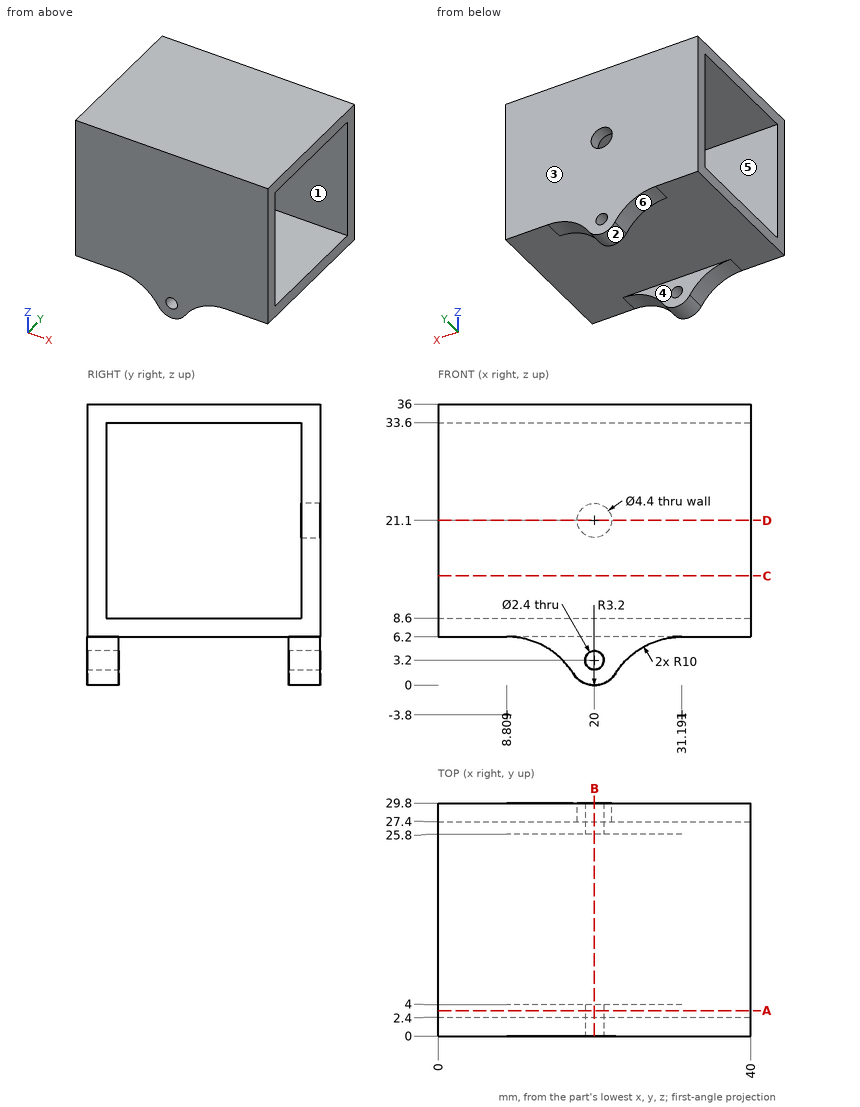
Answer from the drawing. Dimensions are ordinates in mm from the lowest x, y and z of the part. A direction names the side the tool comes from. Coordinates: 2 decimals unless noted, no trailing zeros. Write each loop counter-clockwise with the first axis right and the second up, starting at its lowest first coordinate (ties: lowest second). Pieces come first, ordered by that corner, then holes. Notation, with made-up numbers: M -33,48.25 L -3,48.25 A13 ccw -3,65.25 Z; hole C -8.5,-14.75 d8. An arc over 180 degrees is marked long. Use one line per item in the form item = value. Start each with the question number.
1. The part is cut by section A-A (y = 3.25). Give the vertices of the cut face in (x, z), plus the area to 3 significant figures.
2. Straight lines are drawn through the part: probe 1 along Z at (x, y) = (20, 27.2); probe 2 along Z at (x, y) = (16, 16.25); probe 3 along X at (y, z) = (29.05, 21.1). For each, find the intervals that lie inside material, in ascending order. Write a range as from..to.
3. The part is cut by section B-B (x = 20). Give the vertices of the cut face in (y, z), plus the area to 3 significant figures.
4. The part is cut by section C-C (z = 14). Give the vertices of the cut face in (x, y), plus the area to 3 significant figures.
5. A tool of negligible diameter and unlimited length cuts with its end or side. For the marked faces 5 and 6, from which of +Z, -Z, +X, -X, +Y, -Y can it reach the whole face along a straight path? Write none if from no direction.
6. The mould has two halves that part along Y. Classify the marked faces 1, 2, 3 and 4: released by +Y, released by -Y, zero draft, split by the parting line, or undercut.
7. Each of these flat-tipped pins is pushed along its axis until it touches: P1, Ø5, axis at x = 19, z = 25.5, coming from the -Y side; P2, Ø7.5, axis at x = 17, y = 12.5, coming from the -Z side; P3, Ø2, axis at x = 20, z = 3.2, coming from the +Y side. Where does it stop, or does it pass through?
8. The part is cut by section D-D (z = 21.1). Give the vertices of the cut face in (x, y), plus the area to 3 significant figures.
Evaluation:
q1.outline = M 0,6.2 L 8.81,6.2 A10 cw 17.29,1.5 A3.2 ccw 22.71,1.5 A10 cw 31.19,6.2 L 40,6.2 L 40,8.6 L 0,8.6 Z; M 0,33.6 L 40,33.6 L 40,36 L 0,36 Z; hole C 20,3.2 d2.4
q1.area = 242 mm^2
q2.probe_1 = 0..2, 4.4..8.6, 33.6..36
q2.probe_2 = 6.2..8.6, 33.6..36
q2.probe_3 = 0..17.8, 22.2..40
q3.outline = M 0,0 L 4,0 L 4,2 L 0,2 Z; M 0,4.4 L 4,4.4 L 4,6.2 L 25.8,6.2 L 25.8,4.4 L 29.8,4.4 L 29.8,18.9 L 27.4,18.9 L 27.4,8.6 L 2.4,8.6 L 2.4,33.6 L 27.4,33.6 L 27.4,23.3 L 29.8,23.3 L 29.8,36 L 0,36 Z; M 25.8,0 L 29.8,0 L 29.8,2 L 25.8,2 Z
q3.area = 283 mm^2
q4.outline = M 0,0 L 40,0 L 40,2.4 L 0,2.4 Z; M 0,27.4 L 40,27.4 L 40,29.8 L 0,29.8 Z
q4.area = 192 mm^2
q5.face_5 = +X, -X
q5.face_6 = -Z, -X, +Y, -Y
q6.face_1 = undercut
q6.face_2 = zero draft
q6.face_3 = released by +Y
q6.face_4 = undercut
q7.P1 = 0
q7.P2 = 6.2
q7.P3 = through
q8.outline = M 0,0 L 40,0 L 40,2.4 L 0,2.4 Z; M 0,27.4 L 17.8,27.4 L 17.8,29.8 L 0,29.8 Z; M 22.2,27.4 L 40,27.4 L 40,29.8 L 22.2,29.8 Z
q8.area = 181 mm^2
